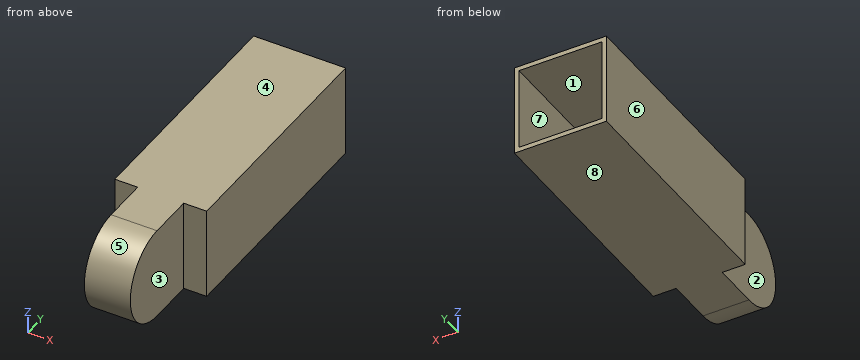
```python
from build123d import *

# Parameters (mm, degrees)
SKETCH_1_W      = 20
SKETCH_1_H      = 20
SKETCH_1_W_2    = 18
SKETCH_1_H_2    = 18
EXTRUDE_1_DEPTH = 50
SKETCH_2_W      = 20
SKETCH_2_H      = 20
EXTRUDE_2_DEPTH = 2
EXTRUDE_3_DEPTH = 5


with BuildPart() as part:
    # 草图1 → 凸台-拉伸1 (new body)
    with BuildSketch(Plane(origin=(0, 0, 0), x_dir=(1, 0, 0), z_dir=(0, 1, 0))):
        Rectangle(SKETCH_1_W, SKETCH_1_H)
        Rectangle(SKETCH_1_W_2, SKETCH_1_H_2, mode=Mode.SUBTRACT)
    extrude(amount=EXTRUDE_1_DEPTH)

    # 草图2 → 凸台-拉伸2 (add)
    with BuildSketch(Plane.XZ):
        Rectangle(SKETCH_2_W, SKETCH_2_H)
    extrude(amount=EXTRUDE_2_DEPTH)

    # 草图6 → 凸台-拉伸3 (add, symmetric)
    with BuildSketch(Plane(origin=(0, 0, 0), x_dir=(0, 0, -1), z_dir=(1, 0, 0))):
        with BuildLine():
            Line((-10, -2), (10, -2))
            Line((10, -2), (10, -12))
            ThreePointArc((10, -12), (0, -22), (-10, -12))
            Line((-10, -12), (-10, -2))
        make_face()
    extrude(amount=EXTRUDE_3_DEPTH, both=True)


solid = part.part
```
Here's how the part is built. I have some questions about the finished solid (model axes, mm). Face numbers are marked on the shaded views. A direction names the side the tool comes from. Coordinates: 2 decimals unless noted, no trailing zeros. Order: outer loops, then holes, each group sorted by start corner. A loop starts at its lowest first (then second) coordinate and runs counter-clockwise, first axis right, second up.
Item 1: Thinking about a two-plate mould opening in Z: for the marked faces 6, 7 and 8, which applies, pulls with the +Z half, pulls with the -Z half, needs draft (parallel to the pull), parting line crosses it, or undercut?
Response values:
face 6: needs draft
face 7: undercut
face 8: pulls with the -Z half
Item 2: Which directions (+Z, -Z, +X, -X, +Y, -Y) give clear straight access to the entire face, cutting with the end or side of a thin tool? Please do the marked faces 1, 2, 3, 4 and 5.
Response values:
face 1: +Y
face 2: +Z, -Z, -X, -Y
face 3: +Z, -Z, +X, -Y
face 4: +Z, +X, -X, +Y, -Y
face 5: +X, -X, -Y
Item 3: If we section it at D-D, the plane x = -7.5: List the corners of the cut face in (y, z) for me.
Response values:
outline: (-2, -10) - (50, -10) - (50, -9) - (0, -9) - (0, 9) - (50, 9) - (50, 10) - (-2, 10) - close
Item 4: If we section it at C-C, the plane x = -1: List the corners of the cut face in (y, z) for me, then the cut area to 3 significant figures.
Response values:
outline: (-12, -10) - (50, -10) - (50, -9) - (0, -9) - (0, 9) - (50, 9) - (50, 10) - (-12, 10) arc R10 ccw to start
area: 497 mm2
Item 5: If we section it at A-A, the plane y = 15.5: List the corners of the cut face in (x, z) for me.
Response values:
outline: (-10, -10) - (10, -10) - (10, 10) - (-10, 10) - close; hole (-9, -9) - (9, -9) - (9, 9) - (-9, 9) - close
Item 6: I need wall thicknesses on probe 1 along X at (y, z) = (1, -8.75); probe 2 along Y at (x, z) = (7.5, -0.75). Which ranges of each line are inside material? Lowest first, please.
Response values:
probe 1: x = -10 to -9, 9 to 10
probe 2: y = -2 to 0
Item 7: I'm going to push flat-ended pins straight in: pin 1 Ø2 at (x, z) = (-2.5, 3.5) entering from +Y; pin 2 Ø5.5 at (x, z) = (8, 4) entering from -Y; pin 3 Ø6 at (y, z) = (-11.5, -2) entering from -X. Where does each tip first touch, or does it pass through?
Response values:
pin 1: stops at y = 0
pin 2: stops at y = -2
pin 3: stops at x = -5
Item 8: If we section it at B-B, the plane z = 0: List the corners of the cut face in (x, y) for me.
Response values:
outline: (-10, -2) - (-5, -2) - (-5, -22) - (5, -22) - (5, -2) - (10, -2) - (10, 50) - (9, 50) - (9, 0) - (-9, 0) - (-9, 50) - (-10, 50) - close
